Geometry: final body of the model. Coordinates: model frame, mm. A direction names the side the tool comes from. Give positions to 0.01 mm unless a question says otherwise; leave off trailing zeros. Loops run counter-clockwise (first coordinate to the right, second up) from the corner with the lowest first, then second, coordinate; pieces in that order, holes last. Notation, with made-up numbers: (47.25, 75) -> (73.25, 75) arc R36 ccw to (73.25, 113) -> close; hole circle Ø2 at (12, 59.5). An arc over 180 degrees is marked (long way). Answer in a Markdown table with one row per item. Add a question column.
1) Line query: line 1 (Z direction, x = 0, y = 1.1); line 2 (Y direction, x = -0.75, z = -1.6); line 3 (X direction, y = 1, z = -1.1). Output: solid intervals per line, ascending. Write a range as from..to.
2) Section query C-C (y = 9). Return the cut outline in (x, z).
3) Access query for faces 1 (the flat face through (0, 9.95, 0)), 2 (the cylindrical face through (-1.4, 2.46, -0.06)), 3 (the cylindrical face through (-1.45, 7.85, -0.06)). Directions: +Z, -Z, +X, -X, +Y, -Y. A direction counts if a zero-diameter tool reaches every point of the face in a straight line with its end or side. Return the directions, or none.
4) Section query A-A (y = 4). Return the cut outline in (x, z).
5) Section query B-B (x = 0). Return the cut outline in (y, z).
6) First-contact query: P1, Ø1.5, axis at y = 1.5, z = 2, coming from the -X side; P2, Ø2.5, axis at x = 0, z = 0, coming from the -Y side. Flat tips, straight axial feed; report the tip coordinate or a pass-through.
7) Draft query along Z for faces 4 (the flat face through (-2, 6, 0)), 5 (the flat face through (0, 5, 0)), 6 (the flat face through (0, 3, 2.85)). Return one class per face: +Z half, -Z half, draft (parallel to the pull), parting line (faces both ways), or undercut.
```python
from build123d import *

# Parameters (mm, degrees)
SKETCH1_R           = 1.4
BOSS_EXTRUDE1_DEPTH = 5
BOSS_EXTRUDE2_DEPTH = 1
SKETCH3_R           = 1.45
BOSS_EXTRUDE3_DEPTH = 3.95
CHAMFER1_SIZE       = 0.2


with BuildPart() as part:
    # Sketch1 → Boss-Extrude1 (new body)
    with BuildSketch(Plane(origin=(0, 0, 0), x_dir=(1, 0, 0), z_dir=(0, 1, 0))):
        Polygon((1.645448267, -2.85), (3.290896534, 0), (1.645448267, 2.85), (-1.645448267, 2.85), (-3.290896534, 0), (-1.645448267, -2.85), align=None)
        Circle(SKETCH1_R, mode=Mode.SUBTRACT)
    extrude(amount=BOSS_EXTRUDE1_DEPTH)

    # Sketch2 → Boss-Extrude2 (add)
    with BuildSketch(Plane(origin=(0, 5, 0), x_dir=(1, 0, 0), z_dir=(0, 1, 0))):
        Polygon((-1.645448267, -2.85), (1.645448267, -2.85), (3.290896534, 0), (1.645448267, 2.85), (-1.645448267, 2.85), (-3.290896534, 0), align=None)
    extrude(amount=BOSS_EXTRUDE2_DEPTH)

    # Sketch3 → Boss-Extrude3 (add)
    with BuildSketch(Plane(origin=(0, 6, 0), x_dir=(1, 0, 0), z_dir=(0, 1, 0))):
        Circle(SKETCH3_R)
    extrude(amount=BOSS_EXTRUDE3_DEPTH)

    # Chamfer1
    chamfer1_edges = [part.edges().sort_by_distance(p)[0] for p in [
        (-1.45, 9.95, 0),
    ]]
    chamfer(chamfer1_edges, length=CHAMFER1_SIZE)


solid = part.part
```
Evaluation:
| question | item | result |
|---|---|---|
| 1 | line 1 | -2.85..-1.4, 1.4..2.85 |
| 1 | line 2 | 0..6 |
| 1 | line 3 | -2.66..-0.87, 0.87..2.66 |
| 2 | outline | circle Ø2.9 at (0, 0) |
| 3 | face 1 | +Z, -Z, +X, -X, +Y |
| 3 | face 2 | -Y |
| 3 | face 3 | +Y |
| 4 | outline | (-3.29, 0) -> (-1.65, -2.85) -> (1.65, -2.85) -> (3.29, 0) -> (1.65, 2.85) -> (-1.65, 2.85) -> close; hole circle Ø2.8 at (0, 0) |
| 5 | outline | (0, -2.85) -> (6, -2.85) -> (6, -1.45) -> (9.75, -1.45) -> (9.95, -1.25) -> (9.95, 1.25) -> (9.75, 1.45) -> (6, 1.45) -> (6, 2.85) -> (0, 2.85) -> (0, 1.4) -> (5, 1.4) -> (5, -1.4) -> (0, -1.4) -> close |
| 6 | P1 | x = -2.57 |
| 6 | P2 | y = 5 |
| 7 | face 4 | draft |
| 7 | face 5 | undercut |
| 7 | face 6 | +Z half |
